```python
from build123d import *

# Parameters (mm, degrees)
SALIENTE_EXTRUIR1_DEPTH = 2
CROQUIS2_R              = 1
CORTAR_EXTRUIR1_DEPTH   = 2


with BuildPart() as part:
    # Croquis1 → Saliente-Extruir1 (new body)
    with BuildSketch(Plane.XY):
        with BuildLine():
            Line((0, 2), (34, 2))
            ThreePointArc((34, 2), (36, 0), (34, -2))
            Line((34, -2), (0, -2))
            ThreePointArc((0, -2), (-2, 0), (0, 2))
        make_face()
    extrude(amount=SALIENTE_EXTRUIR1_DEPTH)

    # Croquis2 → Cortar-Extruir1 (cut)
    with BuildSketch(Plane.XY.offset(2)):
        Circle(CROQUIS2_R)
        with Locations((16, 0)):
            Circle(CROQUIS2_R)
        with Locations((32, 0)):
            Circle(CROQUIS2_R)
    extrude(amount=-CORTAR_EXTRUIR1_DEPTH, mode=Mode.SUBTRACT)


solid = part.part
```
Check sheet for the modelled part. Datum: model origin and axes. Units: mm. Give positions to 0.01 mm unless a question says otherwise; leave off trailing zeros. Order: outer loops, then holes, each group sorted by start corner. A loop starts at its lowest first (then second) coordinate and runs counter-clockwise, first axis right, second up. Notation, with made-up numbers: M 33,-3 L 79,-3 A20 ccw 79,13 Z; hole C 17,89 d5. An arc over 180 degrees is marked long. Answer in a Markdown table with one row per item. Add a question column.
Q1. Gauge pin test, flat end, axial feed: pin 1 Ø1.2 at (x, y) = (16, 0) entering from +Z. Record the tip position at first contact, or that the pin passes through.
Q2. Sectioned sample at C-C, the plane z = 0.75. Record the boundary of the cut face in (x, y).
Q3. Thickness scan on L1, parallel to Y at x = 32, z = 1.35; L2, parallel to X at y = 0.5, z = 0.8; L3, parallel to X at y = -0.4, z = 0.8. Record the ranges inside material, lowest first.
Q4. Sectioned sample at B-B, the plane y = 0. Record the boundary of the cut face in (x, z), and give its area (3 significant figures).
Q5. Sectioned sample at A-A, the plane x = 16. Record the boundary of the cut face in (y, z), and give its area (3 significant figures).
Verdict:
| question | item | result |
|---|---|---|
| 1 | pin 1 | through |
| 2 | outline | M 0,-2 L 34,-2 A2 ccw 34,2 L 0,2 A2 ccw Z; hole C 0,0 d2; hole C 16,0 d2; hole C 32,0 d2 |
| 3 | L1 | -2 to -1, 1 to 2 |
| 3 | L2 | -1.94 to -0.87, 0.87 to 15.13, 16.87 to 31.13, 32.87 to 35.94 |
| 3 | L3 | -1.96 to -0.92, 0.92 to 15.08, 16.92 to 31.08, 32.92 to 35.96 |
| 4 | outline | M -2,0 L -1,0 L -1,2 L -2,2 Z; M 1,0 L 15,0 L 15,2 L 1,2 Z; M 17,0 L 31,0 L 31,2 L 17,2 Z; M 33,0 L 36,0 L 36,2 L 33,2 Z |
| 4 | area | 64.0 mm² |
| 5 | outline | M -2,0 L -1,0 L -1,2 L -2,2 Z; M 1,0 L 2,0 L 2,2 L 1,2 Z |
| 5 | area | 4.00 mm² |
